Autodesk Inventor part; units mm, degrees
ref_plane "YZ Plane" through (0, 0, 0) normal (1, 0, 0) x (0, 1, 0)
ref_plane "XZ Plane" through (0, 0, 0) normal (0, 1, 0) x (-1, 0, 0)
ref_plane "XY Plane" through (0, 0, 0) normal (0, 0, 1) x (1, 0, 0)
sketch "Sketch1" plane through (0, 0, 0) normal (0, 0, 1) x (1, 0, 0)
  line L0 (1200, 2950) -> (-1200, 2950)
  line L1 (-1200, 2950) -> (-1200, 0)
  line L2 (-1200, 0) -> (1200, 0)
  line L3 (1200, 0) -> (1200, 2950)
  line L4 (1150, 2950) -> (1150, 0)
  line L5 (-1150, 0) -> (-1150, 2950) construction
  line L6 (0, 2950) -> (0, 50) construction
  line L7 (-1100, 200) -> (-950, 50)
  line L8 (-1200, 100) -> (-1100, 100)
  line L9 (-1100, 100) -> (-1100, 0)
  line L10 (-1100, 200) -> (-1150, 2950)
  arc A0 (-1100.4545, 224.9959) -> (-1082.3223, 182.3223) centre (-1100, 200) ccw
  arc A1 (-1082.3223, 182.3223) -> (-1100.4545, 224.9959) centre (-1100, 200) ccw construction
  line L11 (-1200, 255) -> (-1101, 255) construction
  line L12 (0, 50) -> (-950, 50)
  line L13 (0, 50) -> (0, 0)
  line L14 (1505.3449, -225.894) -> (355.3449, -225.894)
  line L15 (-1200, 245) -> (-1100.8182, 245)
  line L16 (-1200, 2900) -> (-1149.0909, 2900)
  line L17 (-1115.5511, 1055.3131) -> (-403, 264.2623)
  line L18 (-1200, 1174.3582) -> (-1117.7156, 1174.3582)
  line L19 (-403, 0) -> (-403, 264.2623)
  line L20 (-453, 0) -> (-453, 319.7706)
  line L21 (-1200, 1074.3582) -> (-403, 189.555)
  line L22 (-453, 53) -> (-403, 53)
  line L23 (-1200, 245) -> (-101.8902, 245) construction
  point P0 (-453, 245.0633)
  point P1 (-453, 50)
  point P2 (-403, 50)
  dimension "d3" = 2400
  dimension "d4" = 2950
  dimension "d5" = 50
  dimension "d6" = 100
  dimension "d7" = 50
  dimension "d9" = 135
  dimension "d10" = 950
  dimension "d11" = 1150
  dimension "d12" = 136.042
  dimension "d13" = 50
  dimension "d14" = 100
  dimension "d15" = 212.132
  dimension "d17" = 55
  dimension "d20" = 200
  dimension "d50" = 2705
  dimension "d53" = 50
  dimension "d55" = 1895
  dimension "d57" = 100
  dimension "d59" = 403
  dimension "d60" = 50
  dimension "d62" = 50
  dimension "d63" = 3
  dimension "d65" = 264.2623
extrude "Plate1" add sketch "Sketch1" along normal blind 3 contours L10 L21 L1 L18 | L17 L20 L21 L10 | L17 L19 L21 L20 | L22 L20 L21 L19
equation "\"d11\" = d10 + d18"
equation "\"d14\" = d6"
equation "\"d2\" = Thickness"
equation "\"BendReliefWidth\" = Thickness"
equation "\"BendReliefDepth\" = 0.5 * Thickness"
equation "\"CornerReliefSize\" = 4 * Thickness"
equation "\"MinimumRemnant\" = 2 * Thickness"
equation "\"TransitionRadius\" = BendRadius"
equation "\"JacobiRadiusSize\" = BendRadius"
equation "\"GapSize\" = Thickness"
equation "\"d18\" = d19"
properties part number "BSH 025 rib board cone" material "09g2s"
For this review, take the finished solid that the model builds, in its own axes (mm). Coordinates: 2 decimals unless noted, no trailing zeros. Loops run counter-clockwise (first coordinate to the right, second up) from the corner with the lowest first, then second, coordinate; pieces in that order, holes last. Notation, with made-up numbers: (81.25, 89.5) - (140.25, 89.5) arc R23 cw to (140.25, 123.5) - close; hole circle Ø2 at (-34.75, -7.75). An arc over 180 degrees is marked (long way). Use one line per item in the form item = value. Start each with the question number.
1) For pin 1 (1.5 mm diameter, centred on y = 578, z = 1.5, fed in from -X); pin 2 (1 mm diameter, centred on x = -1034, z = 1, fed in from -Y), all flat-tipped, find the tip position at first contact; note any pin that passes through.
2) To check wall thickness, follow probe 1 along X at (y, z) = (200, 2.1); probe 2 along X at (y, z) = (734, 0.85); probe 3 along Y at (x, z) = (-989.5, 2.2). State the ranges of each line that lie inside material, in increasing order. Write a range as from..to.
3) Take a section at A-A (z = 2.15). State the section outline as (x, y) points, plus the area to 3 significant figures.
4) Take a section at C-C (x = -918). State the section outline as (y, z) points.
5) Draft analysis for pull direction Z (two halves, no side actions). For faces 1 (the face through (-831.729, 665.516, 1.479)), 2 (the face through (-803, 658, 0)), 3 (the face through (-803, 658, 3)), state which applies: released by +Z, released by -Z, zero draft, split by the parting line, or undercut.
6) Take a section at B-B (y = 1103). State the section outline as (x, z) points, plus the area to 3 significant figures.
From the geometry:
q1.pin_1 = -753.57
q1.pin_2 = 889.52
q2.probe_1 = -453..-403
q2.probe_2 = -893.42..-826.12
q2.probe_3 = 840.67..915.38
q3.outline = (-1200, 1074.36) - (-453, 245.06) - (-453, 53) - (-403, 53) - (-403, 264.26) - (-1115.55, 1055.31) - (-1117.72, 1174.36) - (-1200, 1174.36) - close
q3.area = 73,700 mm2
q4.outline = (761.29, 0) - (836, 0) - (836, 3) - (761.29, 3) - close
q5.face_1 = zero draft
q5.face_2 = released by -Z
q5.face_3 = released by +Z
q6.outline = (-1200, 0) - (-1116.42, 0) - (-1116.42, 3) - (-1200, 3) - close
q6.area = 251 mm2
